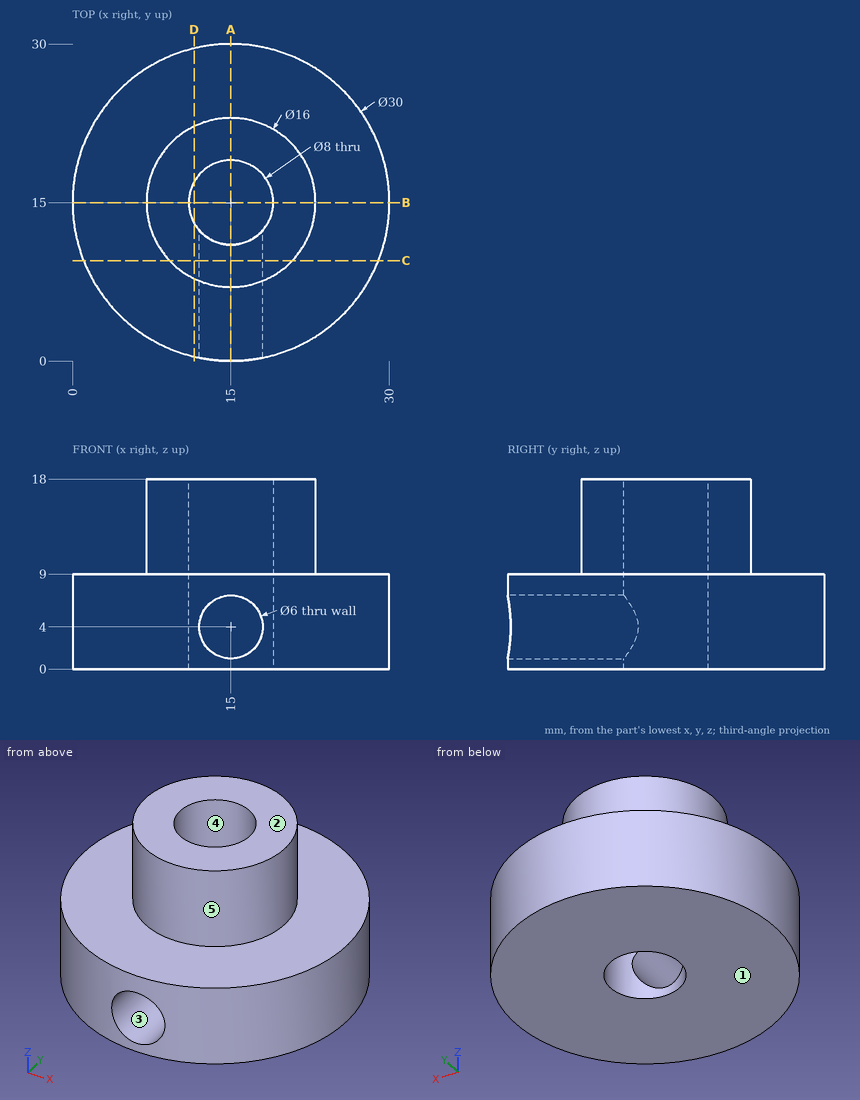
Study the drawing (mm; zero at the part's minimum x, y, z) and answer. A direction names the side the tool comes from. Round coordinates to 2 decimals unless told otherwise and drop trailing zeros. Order: outer loops, then holes, each group sorted by start corner. A loop starts at its lowest first (then second) coordinate and runs counter-clockwise, first axis right, second up. Notation, with made-up numbers: (48.5, -25) -> (95.5, -25) arc R24 cw to (95.5, 5) -> close; hole circle Ø8 at (11.5, 69.25). An arc over 180 degrees is marked (long way). Write each question's results on one line, items separated by ' | '. Start each with the question number.
Q1. Find section A-A (x = 15). Determine the outline of the cut face in (y, z), then the cut area to 3 significant figures.
Q2. Find section C-C (y = 9.5). Determine the outline of the cut face in (x, z), then the cut area to 3 significant figures.
Q3. Find section D-D (x = 11.5). Determine the outline of the cut face in (y, z), then the cut area to 3 significant figures.
Q4. Which of the six approach directions +Z, -Z, +X, -X, +Y, -Y give full straight-line access (tool end or side, diameter ignored) to the marked faces 4 and 5?
Q5. Straight lines are drawn through the part: probe 1 along Y at (x, z) = (15, 8); probe 2 along Y at (x, z) = (15, 10); probe 3 along Z at (x, y) = (12.5, 27). For each, find the intervals that lie inside material, in ascending order. Write a range as from..to.
Q6. The mould has two halves that part along Z. Classify the marked faces 1, 2 and 3: pulls with the +Z half, pulls with the -Z half, needs draft (parallel to the pull), parting line crosses it, or undercut.
Q7. Find section B-B (y = 15). Determine the outline of the cut face in (x, z), then the cut area to 3 significant figures.
Q8. Each of these flat-tipped pins is pushed along its axis until it touches: pin 1 (6 mm diameter, centred on x = 24, z = 5.5, fed in from -Y); pin 2 (5 mm diameter, centred on x = 15, z = 4, fed in from -Y); pin 3 (5 mm diameter, centred on x = 24.5, z = 6, fed in from +Y). Where does it stop, or does it pass through?
Worked answers:
1) outline: (0, 0) -> (11, 0) -> (11, 1) -> (0, 1) -> close; (0, 7) -> (11, 7) -> (11, 18) -> (7, 18) -> (7, 9) -> (0, 9) -> close; (19, 0) -> (30, 0) -> (30, 9) -> (23, 9) -> (23, 18) -> (19, 18) -> close | area: 204 mm2
2) outline: (1.04, 0) -> (28.96, 0) -> (28.96, 9) -> (20.81, 9) -> (20.81, 18) -> (9.19, 18) -> (9.19, 9) -> (1.04, 9) -> close; hole circle Ø6 at (15, 4) | area: 327 mm2
3) outline: (0.41, 0) -> (13.06, 0) -> (13.06, 18) -> (7.81, 18) -> (7.81, 9) -> (0.41, 9) -> close; (16.94, 0) -> (29.59, 0) -> (29.59, 9) -> (22.19, 9) -> (22.19, 18) -> (16.94, 18) -> close | area: 322 mm2
4) face 4: +Z, -Z | face 5: +Z
5) probe 1: y = 0..11, 19..30 | probe 2: y = 7..11, 19..23 | probe 3: z = 0..9
6) face 1: pulls with the -Z half | face 2: pulls with the +Z half | face 3: undercut
7) outline: (0, 0) -> (11, 0) -> (11, 18) -> (7, 18) -> (7, 9) -> (0, 9) -> close; (19, 0) -> (30, 0) -> (30, 9) -> (23, 9) -> (23, 18) -> (19, 18) -> close | area: 270 mm2
8) pin 1: stops at y = 1.25 | pin 2: stops at y = 18.12 | pin 3: stops at y = 28.27
